Read the model definition and answer for the solid it produces. Units are mm, in the model's axes. A direction names the side the tool comes from. Round coordinates to 2 decimals unless told otherwise and drop trailing zeros. Order: outer loops, then holes, each group sorted by start corner. A loop starts at its lowest first (then second) coordinate and runs counter-clockwise, first axis right, second up. Notation, with made-up numbers: (-27, -14) -> (16, -14) arc R20 ccw to (16, -4) -> close; hole circle Ø3 at (-13, 10). An arc over 180 degrees is marked (long way). Answer as a JSON object with one key per item and string values. Group by question number.
Item 1: Consider probe 1 along X at (y, z) = (-22.5, 50); probe 2 along Y at (x, z) = (1.5, 24.5); probe 3 along Z at (x, y) = (-0.75, -13). Determine where each line is inside the solid, lowest interval first. Write a range as from..to.
Item 2: Given P1, Ø1.5, axis at x = 0, z = -29, coming from the -Y side; P2, Ø1.5, axis at x = 3, y = -24, coming from the +Z side; P3, Ø1.5, axis at x = 3, y = -8.5, coming from the +Z side, each flat-ended and moving along its own axis, determine where each tip first touches the part or whether it passes through.
Item 3: For faces 1 (the cylindrical face through (-0.444, -0.275, 41.139)), 2 (the cylindrical face through (-0.44, -34.01, -27.99)), determine the directions among +Z, -Z, +X, -X, +Y, -Y from which every point of the face is accessible in a straight line to the end or side of a thin tool.
Item 4: Section A-A, the plane x = 2 is taken. Write down the section's boundary in (y, z).
from build123d import *

# Parameters (mm, degrees)
BOSS_EXTRUDE1_DEPTH = 4.5
FILLET2_R           = 1
SHELL1_T            = -0.5


with BuildPart() as part:
    # Sketch1 → Boss-Extrude1 (new, symmetric)
    with BuildSketch(Plane(origin=(0, 0, 0), x_dir=(0, 0, -1), z_dir=(1, 0, 0))):
        with BuildLine():
            Line((-40.125843709, 0), (40.125843709, 0))
            ThreePointArc((40.125843709, 0), (44.455970728, -2.5), (44.455970728, -7.5))
            Line((44.455970728, -7.5), (29.896385384, -32.717941552))
            ThreePointArc((29.896385384, -32.717941552), (28.231372637, -34.448445768), (25.95158068, -35.203072113))
            Line((25.95158068, -35.203072113), (-23.293348854, -39.009425834))
            ThreePointArc((-23.293348854, -39.009425834), (-23.94733545, -39.017072006), (-24.596725125, -38.939290383))
            Line((-24.596725125, -38.939290383), (-53.005406797, -33.632936662))
            ThreePointArc((-53.005406797, -33.632936662), (-56.629531724, -30.808063795), (-56.41747986, -26.217941552))
            Line((-56.41747986, -26.217941552), (-41.857894516, -1))
            ThreePointArc((-41.857894516, -1), (-41.125843709, -0.267949192), (-40.125843709, 0))
        make_face()
    extrude(amount=BOSS_EXTRUDE1_DEPTH, both=True)

    # Fillet2
    fillet2_edges = [part.edges().sort_by_distance(p)[0] for p in [
        (4.5, -30.808063795, 56.629531724),
        (4.5, -36.286113523, 38.801065961),
        (4.5, -39.017072006, 23.94733545),
        (4.5, -37.106248974, -1.329115913),
        (4.5, -34.448445768, -28.231372637),
        (4.5, -20.108970776, -37.176178056),
        (4.5, -2.5, -44.455970728),
        (4.5, 0, 0),
        (4.5, -0.267949192, 41.125843709),
        (4.5, -13.608970776, 49.137687188),
    ]]
    fillet(fillet2_edges, radius=FILLET2_R)

    # Shell1
    shell1_openings = [part.faces().sort_by_distance(p)[0] for p in [
        (-4.5, -18.296225023, 6.473740626),
    ]]
    offset(amount=SHELL1_T, openings=shell1_openings, kind=Kind.INTERSECTION)


solid = part.part
Values found:
{
 "1": {"probe 1": "4..4.5", "probe 2": "-38.96..-38.45, -0.5..0", "probe 3": "-41.28..-40.7, 48.21..48.79"},
 "2": {"P1": "y = -34.44", "P2": "z = 55.57", "P3": "z = 46.62"},
 "3": {"face 1": "+Z, +X, -X, +Y", "face 2": "-X"},
 "4": {"outline": "(-39.01, 23.29) -> (-35.2, -25.95) arc R5 ccw to (-32.72, -29.9) -> (-7.5, -44.46) arc R5 ccw to (0, -40.13) -> (0, 40.13) arc R2 ccw to (-1, 41.86) -> (-26.22, 56.42) arc R5 ccw to (-33.63, 53.01) -> (-38.94, 24.6) arc R5 ccw to start; hole (-38.51, 23.33) -> (-34.7, -25.91) arc R4.5 ccw to (-32.47, -29.46) -> (-7.25, -44.02) arc R4.5 ccw to (-0.5, -40.13) -> (-0.5, 40.13) arc R1.5 ccw to (-1.25, 41.42) -> (-26.47, 55.98) arc R4.5 ccw to (-33.14, 52.91) -> (-38.45, 24.5) arc R4.5 ccw to start"}
}
